The model under review builds one solid part; all positions refer to its coordinate system, in mm. A direction names the side the tool comes from. Coordinates: 2 decimals unless noted, no trailing zeros. Answer in a Markdown table with one row per item.
from build123d import *

# Parameters (mm, degrees)
SKETCH1_W           = 2
SKETCH1_H           = 10
BOSS_EXTRUDE1_DEPTH = 100
SKETCH3_R           = 2.15
CUT_EXTRUDE1_DEPTH  = 90
FILLET1_R           = 5
CUT_EXTRUDE2_DEPTH  = 90
FILLET2_R           = 5
BOSS_EXTRUDE2_START = 0.7
SKETCH5_R           = 3.15
SKETCH5_R_2         = 2.15
BOSS_EXTRUDE2_DEPTH = 0.7


# Some blends are built 0.0001 mm under size
with BuildPart() as part:
    # Sketch1 → Boss-Extrude1 (new body)
    with BuildSketch(Plane(origin=(0, 0, 0), x_dir=(1, 0, 0), z_dir=(0, 1, 0))):
        with Locations((1, 5)):
            Rectangle(SKETCH1_W, SKETCH1_H)
    extrude(amount=BOSS_EXTRUDE1_DEPTH)

    # Sketch3 → Cut-Extrude1 (cut)
    with BuildSketch(Plane(origin=(2, 0, 0), x_dir=(0, 0, -1), z_dir=(1, 0, 0))):
        with Locations((5, 5)):
            Circle(SKETCH3_R)
    extrude(amount=-CUT_EXTRUDE1_DEPTH, mode=Mode.SUBTRACT)

    # Fillet1
    fillet1_edges = [part.edges().sort_by_distance(p)[0] for p in [
        (1, 0, -10),
        (1, 0, 0),
    ]]
    fillet(fillet1_edges, radius=FILLET1_R - 0.0001)  # a hair under: the kernel refuses the full size

    # Sketch4 → Cut-Extrude2 (cut)
    with BuildSketch(Plane.ZY):
        with BuildLine():
            add(Edge.make_bspline(
                [(-10, 5), (-7.336619142, 42.407665675), (-7.11394722, 65.464300782), (-10, 100)],
                knots=[0, 0, 0, 0, 1, 1, 1, 1], degree=3))
            Line((-10, 100), (-10, 5))
        make_face()
        with BuildLine():
            add(Edge.make_bspline(
                [(0, 5), (-2.663380858, 42.407665675), (-2.88605278, 65.464300782), (0, 100)],
                knots=[0, 0, 0, 0, 1, 1, 1, 1], degree=3))
            Line((0, 100), (0, 5))
        make_face()
    extrude(amount=-CUT_EXTRUDE2_DEPTH, mode=Mode.SUBTRACT)

    # Fillet2
    # the kernel refuses this fillet: 5 mm, written as the material it takes off along each edge
    with BuildSketch(Plane(origin=(2, 100, -10), x_dir=(0, -0.9968008899824262, 0.07992487554099316), z_dir=(-1, 0, 0)), Plane(origin=(0, 100, 0), x_dir=(0, -0.9968008899824262, -0.07992487554099297), z_dir=(1, 0, 0))) as fillet2_piece_1:
        with BuildLine():
            CenterArc((5.416951327, 4.999969042), FILLET2_R, 175.415752406, 94.382624457)
            Line((0.432946877, 5.39959342), (0.333266788, 5.407585907))
            Line((0.333266788, 5.407585907), (-0.099680089, 0.007992488))
            Line((-0.099680089, 0.007992488), (0.000336329, -0.099999434))
            ThreePointArc((0.000336329, -0.099999434), (2.699681925, -0.095355708), (5.399004527, -0.099999381))
            Line((5.399004527, -0.099999381), (5.399356425, 0))
        make_face()
    extrude(amount=2, mode=Mode.SUBTRACT)

    # Sketch5 → Boss-Extrude2 (add)
    with BuildSketch(Plane(origin=(2, 0, 0), x_dir=(0, 0, -1), z_dir=(1, 0, 0)).offset(BOSS_EXTRUDE2_START)):
        with Locations(Location((5, 5, 0), (0, 0, 180))):
            Circle(SKETCH5_R)
        with Locations((5, 5)):
            Circle(SKETCH5_R_2, mode=Mode.SUBTRACT)
    boss_extrude2 = extrude(amount=-BOSS_EXTRUDE2_DEPTH)

    # Mirror1: Boss-Extrude2 across plane
    add(boss_extrude2.mirror(Plane(origin=(1, 0, 0), x_dir=(0, 0, 1), z_dir=(1, 0, 0))))


solid = part.part
(1) To check wall thickness, follow line 1 (Y direction, x = 2.2, z = -4.75); line 2 (X direction, y = 85.5, z = -3); line 3 (Y direction, x = 1.7, z = -5.75). State the ranges of each line that lie inside material, in increasing order. Write a range as [from, to].
Report:
| item | result |
|---|---|
| line 1 | [1.86, 2.86], [7.14, 8.14] |
| line 2 | [0, 2] |
| line 3 | [0.06, 2.99], [7.01, 99.86] |
(2) The part is to be moulded in two halves that separate along Y. For faces 3 (the cylindrical face through (-0.355, 7.795, -3.546)), 4 (the cylindrical face through (0.976, 6.453, -3.415)), 5 (the cylindrical face through (1, 1, -8)), 6 (the flat face through (-0.7, 7.1, -3.6)), say which applies: +Y half, -Y half, draft (parallel to the pull), parting line (faces both ways), or undercut.
Report:
| item | result |
|---|---|
| face 3 | parting line |
| face 4 | undercut |
| face 5 | -Y half |
| face 6 | draft |
(3) Insertion check: P1, Ø2, axis at x = 1, z = -3.5, coming from the -Y side; P2, Ø2.5, axis at y = 5, z = -5, coming from the +X side; P3, Ø5, axis at y = 51.5, z = -3, coming from the +X side; P4, Ø3, axis at y = 41, z = -7, coming from the -X side. Each pin has a flat end and moves straight along its axis. Give the tip position at first contact, or say it passes through.
Report:
| item | result |
|---|---|
| P1 | y = 0.03 |
| P2 | through |
| P3 | x = 2 |
| P4 | x = 0 |
(4) Machinability: for faces 1 (the cylindrical face through (2.355, 7.795, -3.546)), 2 (the flat face through (2.7, 7.1, -3.6)), which of the approach directions +Z, -Z, +X, -X, +Y, -Y give a long, thin tool a straight path to every point of the face, cutting with its end or side? Answer none if there is none.
Report:
| item | result |
|---|---|
| face 1 | +X |
| face 2 | +Z, -Z, +X, +Y, -Y |
